from build123d import *

# Parameters (mm, degrees)
F0_R     = 10.9
F1_DEPTH = 3


with BuildPart() as f1:
    # F0 (on Top) → F1 (new body)
    with BuildSketch(Plane.XY):
        with BuildLine():
            Line((14.3, 0), (14.3, 25.7))
            ThreePointArc((14.3, 25.7), (0, 40), (-14.3, 25.7))
            Line((-14.3, 25.7), (-14.3, 0))
            Line((-14.3, 0), (-14.3, -25.7))
            ThreePointArc((-14.3, -25.7), (0, -40), (14.3, -25.7))
            Line((14.3, -25.7), (14.3, 0))
        make_face()
        Polygon((0, -14.961285), (9.3, -20.330642), (9.3, -31.069358), (0, -36.438715), (-9.3, -31.069358), (-9.3, -20.330642), align=None, mode=Mode.SUBTRACT)
        Circle(F0_R, mode=Mode.SUBTRACT)
        Polygon((0, 14.961285), (-9.3, 20.330642), (-9.3, 31.069358), (0, 36.438715), (9.3, 31.069358), (9.3, 20.330642), align=None, mode=Mode.SUBTRACT)
    extrude(amount=F1_DEPTH)


solid = f1.part
Could you check a few things on this model? Use its own coordinates, in mm. A direction names the side the tool comes from. Round coordinates to 2 decimals unless told otherwise and drop trailing zeros. Write each loop counter-clockwise with the first axis right and the second up, starting at its lowest first coordinate (ties: lowest second). Pieces come first, ordered by that corner, then holes. Notation, with made-up numbers: (15, -4) - (74, -4) arc R11 cw to (74, 9) - close; hole circle Ø9 at (13.5, -38). An arc over 180 degrees is marked (long way). Use a Markdown table: item, result.
Q1. For faces 1 (the flat face through (-4.715, 33.716, 1.479)), 2 (the flat face through (6.2, 9.4, 3)), which set-ups out of +Z, -Z, +X, -X, +Y, -Y let a thin tool reach every point of the face, with its end or its side?
Output values:
| item | result |
|---|---|
| face 1 | +Z, -Z |
| face 2 | +Z, +X, -X, +Y, -Y |
Q2. Thinking about a two-plate mould opening in Y: for faces 3 (the cylindrical face through (0, -40, 1)), 4 (the flat face through (-4.585, -33.792, 1.479)), 5 (the cylindrical face through (0, 40, 1)), 6 (the flat face through (6.2, 9.4, 0)), which applies, released by +Y, released by -Y, zero draft, split by the parting line, or undercut?
Output values:
| item | result |
|---|---|
| face 3 | released by -Y |
| face 4 | undercut |
| face 5 | released by +Y |
| face 6 | zero draft |
Q3. Please list where these lines run through material, in increasing order: L1, parallel to Y at x = 0, z = 1.5; L2, parallel to X at y = -21, z = 1.8; L3, parallel to Y at x = -8.25, z = 1.15.
Output values:
| item | result |
|---|---|
| L1 | -40 to -36.44, -14.96 to -10.9, 10.9 to 14.96, 36.44 to 40 |
| L2 | -14.3 to -9.3, 9.3 to 14.3 |
| L3 | -37.38 to -31.68, -19.72 to -7.12, 7.12 to 19.72, 31.68 to 37.38 |
Q4. I want a section at D-D (y = 23). List the corners of the cut face in (x, z) for me, plus the area to 3 significant figures.
Output values:
| item | result |
|---|---|
| outline | (-14.3, 0) - (-9.3, 0) - (-9.3, 3) - (-14.3, 3) - close; (9.3, 0) - (14.3, 0) - (14.3, 3) - (9.3, 3) - close |
| area | 30.0 mm2 |
Q5. I want a section at C-C (x = -2.25). List the corners of the cut face in (y, z) for me.
Output values:
| item | result |
|---|---|
| outline | (-39.82, 0) - (-35.14, 0) - (-35.14, 3) - (-39.82, 3) - close; (-16.26, 0) - (-10.67, 0) - (-10.67, 3) - (-16.26, 3) - close; (10.67, 0) - (16.26, 0) - (16.26, 3) - (10.67, 3) - close; (35.14, 0) - (39.82, 0) - (39.82, 3) - (35.14, 3) - close |
Q6. For pin 1 (8 mm diameter, centred on x = 3, y = -25, fed in from -Z), with a flat end and sliding along its axis, tell me the tip position at first contact or that it passes through.
Output values:
| item | result |
|---|---|
| pin 1 | through |
Q7. I want a section at B-B (z = 1.45). List the corners of the cut face in (x, y) for me, plus the area to 3 significant figures.
Output values:
| item | result |
|---|---|
| outline | (-14.3, -25.7) arc R14.3 ccw to (14.3, -25.7) - (14.3, 25.7) arc R14.3 ccw to (-14.3, 25.7) - close; hole circle Ø21.8 at (0, 0); hole (-9.3, -31.07) - (0, -36.44) - (9.3, -31.07) - (9.3, -20.33) - (0, -14.96) - (-9.3, -20.33) - close; hole (-9.3, 20.33) - (0, 14.96) - (9.3, 20.33) - (9.3, 31.07) - (0, 36.44) - (-9.3, 31.07) - close |
| area | 1,140 mm2 |
Q8. I want a section at A-A (y = 0). List the corners of the cut face in (x, z) for me.
Output values:
| item | result |
|---|---|
| outline | (-14.3, 0) - (-10.9, 0) - (-10.9, 3) - (-14.3, 3) - close; (10.9, 0) - (14.3, 0) - (14.3, 3) - (10.9, 3) - close |
